The model under review builds one solid part; all positions refer to its coordinate system, in mm. Face numbers are marked on the shaded views. A direction names the side the tool comes from. Give positions to 0.01 mm unless a question says otherwise; leave off trailing zeros. Order: outer loops, then holes, each group sorted by start corner. A loop starts at its lowest first (then second) coordinate and runs counter-clockwise, first axis right, second up. Notation, with made-up numbers: (79.25, 8) -> (121.25, 8) arc R16 cw to (121.25, 14) -> close; hole circle Ø7 at (-27.75, 26.5). An arc over 180 degrees is marked (long way). Answer as a JSON object with one key per item and string values. Group by question number.
from build123d import *
from OCP.BRepFilletAPI import BRepFilletAPI_MakeChamfer

# Parameters (mm, degrees)
EXTRUDE_1_DEPTH     = 45
CHAMFER_1_SIZE      = 7
CHAMFER_1_SIZE2     = 4.901452767
CUT_EXTRUDE_START   = 13
CUT_EXTRUDE_1_DEPTH = 13
CUT_EXTRUDE_2_DEPTH = 6
CUT_EXTRUDE_3_DEPTH = 6
CHAMFER_START       = -1
CHAMFER_2_DEPTH     = 7
CHAMFER_3_SIZE      = 7
CHAMFER_3_SIZE2     = 4.901452767


with BuildPart() as part:
    # 草图1 → 凸台-拉伸1 (new body)
    with BuildSketch(Plane.XY):
        with BuildLine():
            Line((0, 0), (0, 144.272111773))
            ThreePointArc((0, 144.272111773), (-7.734402303, 154.012084416), (-18.973413415, 148.68548369))
            Line((-18.973413415, 148.68548369), (-38, 110))
            Line((-38, 110), (-38, 33.669600757))
            ThreePointArc((-38, 33.669600757), (-49.996050511, 18.969691065), (-49.617376915, 0))
            Line((-49.617376915, 0), (0, 0))
        make_face()
    extrude(amount=EXTRUDE_1_DEPTH)

    # 草图2 → 切除-旋转2 (revolve, cut)
    with BuildSketch(Plane(origin=(-24, 0, 0), x_dir=(0, 0, -1), z_dir=(1, 0, 0)), mode=Mode.PRIVATE) as cut_revolve_2_sk:
        Polygon((-45, 23), (-45, 10), (0, 10), (0, 15), (-4.3, 15), (-10.3, 15), (-10.3, 12.5), (-14.3, 12.5), (-14.3, 14), (-13.8, 14), (-13.8, 35), (-26.8, 35), (-26.8, 14), (-26.3, 14), (-26.3, 12.5), (-30.8, 12.5), (-30.8, 15), (-35.7, 15), (-35.7, 23), align=None)
    revolve(cut_revolve_2_sk.sketch.rotate(Axis((-24, 10, 45), (0, 0, -1)), 90), axis=Axis((-24, 10, 45), (0, 0, -1)), mode=Mode.SUBTRACT)

    # 倒角1
    chamfer_1_edges = [part.edges().sort_by_distance(p)[0] for p in [
        (-49.996050511, 18.969691065, 45),
        (-49.996050511, 18.969691065, 0),
    ]]
    chamfer_1_side = [part.faces().sort_by_distance(p)[0] for p in [
        (-49.996050511, 18.969691065, 22.5),
    ]]
    chamfer(chamfer_1_edges, length=CHAMFER_1_SIZE, length2=CHAMFER_1_SIZE2, reference=chamfer_1_side[0])

    # 草图4 → 切除-拉伸1 (cut)
    with BuildSketch(Plane.XY.offset(13.8).offset(CUT_EXTRUDE_START)):
        with BuildLine():
            Line((-24, 35), (0, 35))
            Line((0, 35), (0, 17))
            ThreePointArc((0, 17), (-9, 30), (-24, 35))
        make_face()
        with BuildLine():
            Line((-1.087121525, 0), (0, 0))
            Line((0, 0), (0, 3))
            ThreePointArc((0, 3), (-0.495648452, 1.482637832), (-1.087121525, 0))
        make_face()
    extrude(amount=-CUT_EXTRUDE_1_DEPTH, mode=Mode.SUBTRACT)

    # 草图7 → 切除-拉伸2 (cut)
    with BuildSketch(Plane(origin=(0, 0, 0), x_dir=(-1, 0, 0), z_dir=(0, 0, -1))):
        with BuildLine():
            Line((27.95, 1.469792729), (27.95, 4.702830945))
            ThreePointArc((27.95, 4.702830945), (28.032732694, 5.101103075), (28.267241379, 5.433474952))
            ThreePointArc((28.267241379, 5.433474952), (30.25, 10), (28.267241379, 14.566525048))
            ThreePointArc((28.267241379, 14.566525048), (28.032732694, 14.898896925), (27.95, 15.297169055))
            Line((27.95, 15.297169055), (27.95, 18.530207271))
            ThreePointArc((27.95, 18.530207271), (27.928074545, 18.997939916), (27.862490469, 19.46157046))
            Line((27.862490469, 19.46157046), (26.357995425, 27.397054331))
            ThreePointArc((26.357995425, 27.397054331), (24, 29.35), (21.642004575, 27.397054331))
            Line((21.642004575, 27.397054331), (20.137509531, 19.46157046))
            ThreePointArc((20.137509531, 19.46157046), (20.071925455, 18.997939916), (20.05, 18.530207271))
            Line((20.05, 18.530207271), (20.05, 15.297169055))
            ThreePointArc((20.05, 15.297169055), (19.967267306, 14.898896925), (19.732758621, 14.566525048))
            ThreePointArc((19.732758621, 14.566525048), (17.75, 10), (19.732758621, 5.433474952))
            ThreePointArc((19.732758621, 5.433474952), (19.967267306, 5.101103075), (20.05, 4.702830945))
            Line((20.05, 4.702830945), (20.05, 1.469792729))
            ThreePointArc((20.05, 1.469792729), (20.071925455, 1.002060084), (20.137509531, 0.53842954))
            Line((20.137509531, 0.53842954), (21.642004575, -7.397054331))
            ThreePointArc((21.642004575, -7.397054331), (24, -9.35), (26.357995425, -7.397054331))
            Line((26.357995425, -7.397054331), (27.862490469, 0.53842954))
            ThreePointArc((27.862490469, 0.53842954), (27.928074545, 1.002060084), (27.95, 1.469792729))
        make_face()
    extrude(amount=-CUT_EXTRUDE_2_DEPTH, mode=Mode.SUBTRACT)

    # 草图9 → 切除-拉伸3 (cut)
    with BuildSketch(Plane(origin=(0, 0, 0), x_dir=(-1, 0, 0), z_dir=(0, 0, -1))):
        with BuildLine():
            Line((20.137509531, 19.46157046), (19.478101846, 15.983513774))
            ThreePointArc((19.478101846, 15.983513774), (16.508016808, 9.653318796), (20.05, 3.624460807))
            Line((20.05, 3.624460807), (27.95, 3.624460807))
            ThreePointArc((27.95, 3.624460807), (31.491983192, 9.653318796), (28.521898154, 15.983513774))
            Line((28.521898154, 15.983513774), (27.862490469, 19.46157046))
            Line((27.862490469, 19.46157046), (20.137509531, 19.46157046))
        make_face()
    extrude(amount=-CUT_EXTRUDE_3_DEPTH, mode=Mode.SUBTRACT)

    # 倒角2: read off the stored shape, not the designer's step
    # 倒角2 outline → 倒角2 (cut)
    with BuildSketch(Plane.XY.offset(CHAMFER_START)):
        with BuildLine():
            Line((-20.239590839, 0), (-19.257196744, 0))
            Line((-19.257196744, 0), (-20.080386265, 0.919393486))
            ThreePointArc((-20.080386265, 0.919393486), (-20.105277636, 0.728361179), (-20.137509531, 0.53842954))
            Line((-20.137509531, 0.53842954), (-20.239590839, 0))
        make_face()
        with BuildLine():
            Line((-28.742803256, 0), (-27.760409161, 0))
            Line((-27.760409161, 0), (-27.862490469, 0.53842954))
            ThreePointArc((-27.862490469, 0.53842954), (-27.894722364, 0.728361179), (-27.919613735, 0.919393486))
            Line((-27.919613735, 0.919393486), (-28.742803256, 0))
        make_face()
    extrude(amount=CHAMFER_2_DEPTH, mode=Mode.SUBTRACT)

    # 倒角3: one chamfer whose edges measure the first distance from different faces: ONE call of the kernel's chamfer builder (chamfer() names one face for all edges)
    chamfer_3_edges_1 = [part.edges().sort_by_distance(p)[0] for p in [
        (-38, 68.86981309, 45),
    ]]
    chamfer_3_side_1 = [part.faces().sort_by_distance(p)[0] for p in [
        (-18.29172725, 74.905702605, 45),
    ]]
    chamfer_3_edges_2 = [part.edges().sort_by_distance(p)[0] for p in [
        (-38, 68.86981309, 0),
    ]]
    chamfer_3_side_2 = [part.faces().sort_by_distance(p)[0] for p in [
        (-18.531236566, 72.11524923, 0),
    ]]
    chamfer_3 = BRepFilletAPI_MakeChamfer(part.part.solid().wrapped)
    for e in chamfer_3_edges_1:
        chamfer_3.Add(CHAMFER_3_SIZE, CHAMFER_3_SIZE2, e.wrapped, chamfer_3_side_1[0].wrapped)  # the first distance lies on this face
    for e in chamfer_3_edges_2:
        chamfer_3.Add(CHAMFER_3_SIZE, CHAMFER_3_SIZE2, e.wrapped, chamfer_3_side_2[0].wrapped)  # the first distance lies on this face
    add(Compound.cast(chamfer_3.Shape()), mode=Mode.REPLACE)


solid = part.part
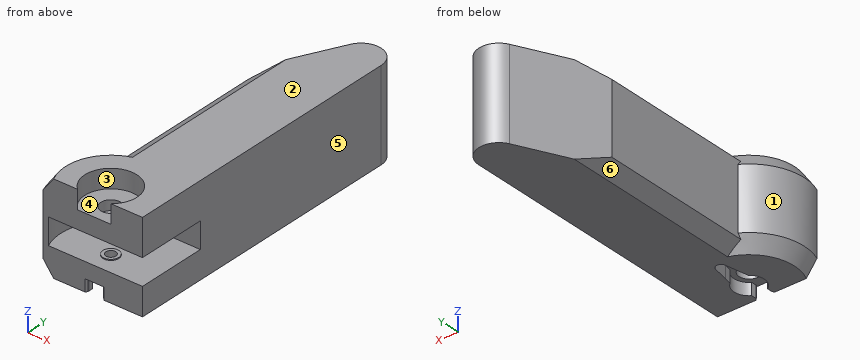
1. Take a section at A-A on z = 23. Give the boundary of the cut face in (x, y).
2. Machinability: for the marked faces 5 and 6, which of the approach directions +Z, -Z, +X, -X, +Y, -Y give a long, thin tool a straight path to every point of the face, cutting with its end or side? Answer none if there is none.
3. Take a section at B-B on y = 52.5. Give the boundary of the cut face in (x, z), plus the area to 3 significant figures.
4. Take a section at C-C on x = -6. Give the boundary of the cut face in (y, z).
5. For probe 1 along X at (y, z) = (61.5, 7); probe 2 along Y at (x, z) = (-24, 11); probe 3 along Y at (x, z) = (-24, 33), list the stretches that pass through material, from the lowest coordinate up. Write a range as [from, to].
6. For pin 1 (2 mm diameter, centred on y = 120.5, z = 23.5, fed in from -X); pin 2 (12 mm diameter, centred on y = 105.5, z = 14, fed in from -X); pin 3 (13 mm diameter, centred on x = -24, y = 10, fed in from -Z), all flat-tipped, find the tip position at first contact; note any pin that passes through.
7. Draft analysis for pull direction Y (two halves, no side actions). For the marked faces 1, 2, 3 and 4, state which applies: pulls with the +Y half, pulls with the -Y half, needs draft (parallel to the pull), parting line crosses it, or undercut.
8. Take a section at D-D on y = 10. State how many separate pieces and enclosed holes the cut face has, plus the area to 3 significant figures.
Checks:
{
 "1": {"outline": "(-49.62, 0) -> (-46.91, 0) arc R25 cw to (-24, 35) -> (0, 35) -> (0, 144.27) arc R10 ccw to (-18.97, 148.69) -> (-38, 110) -> (-38, 33.67) arc R27.5 ccw to start"},
 "2": {"face 5": "+Z, -Z, +X, +Y, -Y", "face 6": "-Z, -X, +Y"},
 "3": {"outline": "(-38, 4.9) -> (-31, 0) -> (0, 0) -> (0, 45) -> (-31, 45) -> (-38, 40.1) -> close", "area": "1,680 mm2"},
 "4": {"outline": "(0, 0) -> (153.44, 0) -> (153.44, 45) -> (0, 45) -> (0, 26.8) -> (35, 26.8) -> (35, 13.8) -> (0, 13.8) -> close"},
 "5": {"probe 1": "x = [-38, 0]", "probe 2": "y = [0, 7.5], [12.5, 138.47]", "probe 3": "y = [0, 5], [15, 138.47]"},
 "6": {"pin 1": "stops at x = -33.33", "pin 2": "stops at x = -38", "pin 3": "stops at z = 6"},
 "7": {"face 1": "parting line crosses it", "face 2": "needs draft", "face 3": "undercut", "face 4": "undercut"},
 "8": {"separate pieces": "3", "enclosed holes": "0", "area": "1,190 mm2"}
}
